Part model, mm, in its own coordinate system. A direction names the side the tool comes from. Give positions to 0.01 mm unless a question says otherwise; leave off trailing zeros. Write each loop counter-clockwise with the first axis right and the second up, starting at its lowest first coordinate (ties: lowest second). Pieces come first, ordered by that corner, then holes. Notation, with made-up numbers: (-23, 65) - (18, 65) arc R24 ccw to (18, 85) - close; hole circle Ø2 at (45.5, 86.5). An arc over 180 degrees is marked (long way). Answer in a Markdown table with one row per item. Add a question column.
1. Drop flat-ended pins along their axis: pin 1 Ø4 at (x, y) = (15, -15) entering from +Z; pin 2 Ø2 at (x, y) = (-18.5, 23.5) entering from -Z. Give the stop position or say it passes through.
2. Band-saw the part on B-B on x = 25. State how many separate pieces and enclosed holes the cut face has, plus the area to 3 significant figures.
3. Pull direction X, two halves, no side cores. Call faces 4 (the cylindrical face through (23.89, -26.01, 29.58)), 5 (the flat face through (0, 0, 25)), 6 (the flat face through (-30, 7, 30)): released by +X, released by -X, zero draft, split by the parting line, or undercut.
4. Probe line 1 along Y through (x, z) = (-25, 42); line 2 along Y through (x, z) = (19.5, 39); line 3 along Y through (x, z) = (-1.5, 30). List the from-to ranges inside material, lowest first.
5. Band-saw the part on C-C on y = 25. Write the cut outline in (x, z).
6. Which spindle directions (+Z, -Z, +X, -X, +Y, -Y) get a long thin tool onto all of the face, cutting with end or side? Do faces 1 (the flat face through (0, -20, 47)), 2 (the cylindrical face through (-0.42, -20.86, 0.9)), 3 (the flat face through (0, 25, 0)). Say none if no direction does.
7. Band-saw the part on A-A on y = 0. Write the cut outline in (x, z), plus the area to 3 significant figures.
8. Band-saw the part on D-D on y = -18.5. Write the cut outline in (x, z), plus the area to 3 significant figures.
Autodesk Inventor part; units mm, degrees
ref_plane "YZ Plane" through (0, 0, 0) normal (1, 0, 0) x (0, 1, 0)
ref_plane "XZ Plane" through (0, 0, 0) normal (0, 1, 0) x (-1, 0, 0)
ref_plane "XY Plane" through (0, 0, 0) normal (0, 0, 1) x (1, 0, 0)
sketch "Sketch1" plane through (0, 0, 0) normal (0, 0, 1) x (1, 0, 0)
  line L0 (-30, -30) -> (30, -30)
  line L1 (30, -30) -> (30, 30)
  line L2 (30, 30) -> (-30, 30)
  line L3 (-30, 30) -> (-30, -30)
  line L4 (-30, -30) -> (30, 30) construction
  line L5 (30, -30) -> (-30, 30) construction
  line L6 (30, 30) -> (25, 30) construction
  line L7 (25, 30) -> (25, 25) construction
  line L8 (-30, 30) -> (-25, 30) construction
  line L9 (-25, 30) -> (-25, 25) construction
  line L10 (-30, -30) -> (-30, -25) construction
  line L11 (-30, -25) -> (-25, -25) construction
  line L12 (30, -30) -> (30, -25) construction
  line L13 (30, -25) -> (25, -25) construction
  circle A0 centre (-25, 25) radius 1.5
  circle A1 centre (25, 25) radius 1.5
  circle A2 centre (25, -25) radius 1.5
  circle A3 centre (-25, -25) radius 1.5
  point P0 (0, 0)
  dimension "d0" = 60
  dimension "d1" = 60
  dimension "d2" = 5
  dimension "d3" = 5
  dimension "d4" = 5
  dimension "d5" = 5
  dimension "d6" = 5
  dimension "d7" = 5
  dimension "d8" = 5
  dimension "d9" = 5
  dimension "d10" = 3
  dimension "d11" = 3
  dimension "d12" = 3
  dimension "d13" = 3
extrude "Block" add sketch "Sketch1" along normal blind 60
sketch "Sketch2" plane through (30, -30, 0) normal (1, 0, 0) x (0, 0, -1)
  line L0 (0, 0) -> (0, 60) construction
  line L1 (-60, 0) -> (0, 60) construction
  circle A0 centre (-30, 30) radius 1
  point P0 (0, 30)
  dimension "d17" = 2
extrude "Motor Mount" cut sketch "Sketch2" against normal blind 60
sketch "Sketch3" plane through (30, -30, 0) normal (1, 0, 0) x (0, 0, -1)
  line L0 (0, 60) -> (-60, 60) construction
  line L1 (-60, 60) -> (-60, 50) construction
  line L2 (-60, 60) -> (-60, 0) construction
  line L3 (-60, 50) -> (0, 50) construction
  line L4 (0, 60) -> (0, 0) construction
  line L5 (-60, 0) -> (-60, 10) construction
  line L6 (-60, 10) -> (0, 10) construction
  circle A0 centre (-30, 30) radius 1 construction
  line L7 (-30, 30) -> (-25, 30) construction
  line L8 (-30, 30) -> (-35, 30) construction
  line L9 (-35, 30) -> (-35, 10) construction
  line L10 (-25, 30) -> (-25, 10) construction
  line L11 (-25, 30) -> (-25, 50) construction
  line L12 (-35, 30) -> (-35, 50) construction
  line L13 (-60, 50) -> (-35, 50)
  line L14 (-35, 10) -> (-60, 10)
  line L15 (-35, 10) -> (-35, 50)
  line L16 (-25, 50) -> (-25, 10)
  line L17 (0, 10) -> (-25, 10)
  line L18 (-25, 50) -> (0, 50)
  line L19 (0, 50) -> (0, 10)
  line L20 (-60, 10) -> (-60, 50)
  point P0 (0, 30)
  dimension "d20" = 10
  dimension "d21" = 10
  dimension "d22" = 5
  dimension "d23" = 5
extrude "Plastic Savings" cut sketch "Sketch3" against normal blind 60
fillet "Fillets FTW" radius 3 12 edges at (0, -30, 60) (0, -20, 60) (0, 30, 60) (0, 20, 60) (0, 20, 35) (0, -20, 35) (0, -20, 0) (0, -30, 0) (0, -20, 25) (0, 20, 25) (0, 30, 0) (0, 20, 0)
properties part number "60x60IdlerNoMotor"
Values:
| question | item | result |
|---|---|---|
| 1 | pin 1 | stops at z = 35 |
| 1 | pin 2 | stops at z = 0 |
| 2 | separate pieces | 3 |
| 2 | enclosed holes | 1 |
| 2 | area | 1,230 mm² |
| 3 | face 4 | undercut |
| 3 | face 5 | zero draft |
| 3 | face 6 | released by -X |
| 4 | line 1 | y = -30 to -26.5, -23.5 to -20, 20 to 23.5, 26.5 to 30 |
| 4 | line 2 | y = -30 to -20, 20 to 30 |
| 4 | line 3 | y = -30 to -1, 1 to 30 |
| 5 | outline | (-30, 0) - (-26.5, 0) - (-26.5, 60) - (-30, 60) - close; (-23.5, 0) - (23.5, 0) - (23.5, 60) - (-23.5, 60) - close; (26.5, 0) - (30, 0) - (30, 60) - (26.5, 60) - close |
| 6 | face 1 | +Z, +X, -X |
| 6 | face 2 | -Z, +X, -X |
| 6 | face 3 | -Z, +X, -X, +Y, -Y |
| 7 | outline | (-30, 25) - (30, 25) - (30, 29) - (-30, 29) - close; (-30, 31) - (30, 31) - (30, 35) - (-30, 35) - close |
| 7 | area | 480 mm² |
| 8 | outline | (-30, 24.6) - (30, 24.6) - (30, 35.4) - (-30, 35.4) - close |
| 8 | area | 648 mm² |
